```python
from build123d import *

# Parameters (mm, degrees)
F1_DEPTH = 2


with BuildPart() as f1:
    # F0 (on Top) → F1 (new body)
    with BuildSketch(Plane.XY):
        with BuildLine():
            ThreePointArc((-5.066449, 0.370803), (-4.939368, 1.187032), (-4.681679, 1.971873))
            ThreePointArc((-4.681679, 1.971873), (-4.674597, 2.264385), (-4.868556, 2.483458))
            Line((-4.868556, 2.483458), (-5.198977, 2.652007))
            ThreePointArc((-5.198977, 2.652007), (-5.401697, 2.897981), (-5.360275, 3.214024))
            ThreePointArc((-5.360275, 3.214024), (-4.962027, 3.800103), (-4.5, 4.337338))
            Line((-4.5, 4.337338), (-4.5, 6))
            ThreePointArc((-4.5, 6), (-5.964466, 9.535534), (-9.5, 11))
            ThreePointArc((-9.5, 11), (-10.56066, 10.56066), (-11, 9.5))
            Line((-11, 9.5), (-11, 0))
            ThreePointArc((-11, 0), (0, -11), (11, 0))
            Line((11, 0), (11, 9.5))
            ThreePointArc((11, 9.5), (10.56066, 10.56066), (9.5, 11))
            ThreePointArc((9.5, 11), (5.964466, 9.535534), (4.5, 6))
            Line((4.5, 6), (4.5, 4.337338))
            ThreePointArc((4.5, 4.337338), (4.941382, 3.82691), (5.325163, 3.271872))
            ThreePointArc((5.325163, 3.271872), (5.370003, 2.956296), (5.169959, 2.708141))
            Line((5.169959, 2.708141), (4.841382, 2.536025))
            ThreePointArc((4.841382, 2.536025), (4.649807, 2.314864), (4.660055, 2.022447))
            ThreePointArc((4.660055, 2.022447), (4.932869, 1.213755), (5.066449, 0.370803))
            ThreePointArc((5.066449, 0.370803), (5.193058, 0.107016), (5.465382, 0))
            Line((5.465382, 0), (5.836309, 0))
            ThreePointArc((5.836309, 0), (6.128661, -0.126998), (6.235373, -0.42735))
            ThreePointArc((6.235373, -0.42735), (6.155048, -1.085301), (6.005496, -1.731045))
            ThreePointArc((6.005496, -1.731045), (5.802494, -1.976786), (5.484336, -1.996135))
            Line((5.484336, -1.996135), (5.135779, -1.869271))
            ThreePointArc((5.135779, -1.869271), (4.843276, -1.876693), (4.634083, -2.081268))
            ThreePointArc((4.634083, -2.081268), (4.399409, -2.54), (4.119473, -2.972599))
            ThreePointArc((4.119473, -2.972599), (4.046902, -3.256054), (4.186725, -3.51308))
            Line((4.186725, -3.51308), (4.470872, -3.751507))
            ThreePointArc((4.470872, -3.751507), (4.613194, -4.036714), (4.501877, -4.33539))
            ThreePointArc((4.501877, -4.33539), (4.017423, -4.787778), (3.487783, -5.186316))
            ThreePointArc((3.487783, -5.186316), (3.174314, -5.244077), (2.918154, -5.054392))
            Line((2.918154, -5.054392), (2.732691, -4.73316))
            ThreePointArc((2.732691, -4.73316), (2.50385, -4.550828), (2.2121, -4.573075))
            ThreePointArc((2.2121, -4.573075), (1.737462, -4.773639), (1.244949, -4.925089))
            ThreePointArc((1.244949, -4.925089), (1.007156, -5.09558), (0.949054, -5.382351))
            Line((0.949054, -5.382351), (1.013464, -5.747642))
            ThreePointArc((1.013464, -5.747642), (0.939162, -6.057606), (0.661903, -6.214852))
            ThreePointArc((0.661903, -6.214852), (0, -6.25), (-0.661903, -6.214852))
            ThreePointArc((-0.661903, -6.214852), (-0.939162, -6.057606), (-1.013464, -5.747642))
            Line((-1.013464, -5.747642), (-0.949054, -5.382351))
            ThreePointArc((-0.949054, -5.382351), (-1.007156, -5.09558), (-1.244949, -4.925089))
            ThreePointArc((-1.244949, -4.925089), (-1.737462, -4.773639), (-2.2121, -4.573075))
            ThreePointArc((-2.2121, -4.573075), (-2.50385, -4.550828), (-2.732691, -4.73316))
            Line((-2.732691, -4.73316), (-2.918154, -5.054392))
            ThreePointArc((-2.918154, -5.054392), (-3.174314, -5.244077), (-3.487783, -5.186316))
            ThreePointArc((-3.487783, -5.186316), (-4.017423, -4.787778), (-4.501877, -4.33539))
            ThreePointArc((-4.501877, -4.33539), (-4.613194, -4.036714), (-4.470872, -3.751507))
            Line((-4.470872, -3.751507), (-4.186725, -3.51308))
            ThreePointArc((-4.186725, -3.51308), (-4.046902, -3.256054), (-4.119473, -2.972599))
            ThreePointArc((-4.119473, -2.972599), (-4.399409, -2.54), (-4.634083, -2.081268))
            ThreePointArc((-4.634083, -2.081268), (-4.843276, -1.876693), (-5.135779, -1.869271))
            Line((-5.135779, -1.869271), (-5.484336, -1.996135))
            ThreePointArc((-5.484336, -1.996135), (-5.802494, -1.976786), (-6.005496, -1.731045))
            ThreePointArc((-6.005496, -1.731045), (-6.155048, -1.085301), (-6.235373, -0.42735))
            ThreePointArc((-6.235373, -0.42735), (-6.128661, -0.126998), (-5.836309, 0))
            Line((-5.836309, 0), (-5.465382, 0))
            ThreePointArc((-5.465382, 0), (-5.193058, 0.107016), (-5.066449, 0.370803))
        make_face()
    extrude(amount=F1_DEPTH)


solid = f1.part
```
Check sheet for the modelled part. Datum: model origin and axes. Units: mm. A direction names the side the tool comes from. Give positions to 0.01 mm unless a question says otherwise; leave off trailing zeros. Write each loop counter-clockwise with the first axis right and the second up, starting at its lowest first coordinate (ties: lowest second). Pieces come first, ordered by that corner, then holes. Notation, with made-up numbers: (32.5, 28) -> (85.5, 28) arc R18 cw to (85.5, 33) -> close; hole circle Ø6 at (-11, 55). An arc over 180 degrees is marked (long way). Use CSV: the item, a comma, the result in double quotes. Start each with the question number.
Q1. Cross-section at A-A on x = 0. Enter the section's corners in (y, z).
Q2. Tool access check on faces 1 (the cylindrical face through (-4.396, -2.546, 0.986)), 2 (the cylindrical face through (-1.731, -4.776, 0.986)), 3 (the flat face through (2, -5, 0)). Record the directions out of +Z, -Z, +X, -X, +Y, -Y that give a thin tool (end or side, any length) a straight path to the whole face; none if there is none.
Q3. Scan lines: line 1 along X through (y, z) = (6, 1.6); line 2 along Y through (x, z) = (5.75, 0.65); line 3 along X through (y, z) = (1.5, 1.3). Record each from-to range of solid material in increasing order.
Q4. Cross-section at B-B on x = -8.25. Enter the section's corners in (y, z).
Working result:
1,outline,"(-11, 0) -> (-6.25, 0) -> (-6.25, 2) -> (-11, 2) -> close"
2,face 1,"+Z, -Z"
2,face 2,"+Z, -Z, +Y"
2,face 3,"-Z, +X, -X, +Y, -Y"
3,line 1,"x = -11 to -4.5, 4.5 to 11"
3,line 2,"y = -9.38 to -2, 0 to 9.31"
3,line 3,"x = -11 to -4.85, 4.85 to 11"
4,outline,"(-7.28, 0) -> (10.84, 0) -> (10.84, 2) -> (-7.28, 2) -> close"
